Autodesk Inventor part; units mm, degrees
ref_plane "YZ Plane" through (0, 0, 0) normal (1, 0, 0) x (0, 1, 0)
ref_plane "XZ Plane" through (0, 0, 0) normal (0, 1, 0) x (-1, 0, 0)
ref_plane "XY Plane" through (0, 0, 0) normal (0, 0, 1) x (1, 0, 0)
sketch "Sketch1" plane through (0, 0, 0) normal (0, 1, 0) x (-1, 0, 0)
  line L0 (-10.16, 10.16) -> (10.16, 10.16)
  line L1 (10.16, 10.16) -> (10.16, -10.16)
  line L2 (-10.16, -10.16) -> (-10.16, 10.16)
  circle A0 centre (6.9088, -6.9148) radius 1.9304
  circle A1 centre (6.9088, 6.9088) radius 1.9304
  circle A2 centre (-6.9088, 6.9088) radius 1.9304
  circle A3 centre (-6.9088, -6.9148) radius 1.9304
  line L3 (-5.715, -10.16) -> (-5.715, -20.574)
  line L4 (-5.715, -20.574) -> (5.715, -20.574)
  line L5 (5.715, -20.574) -> (5.715, -10.16)
  line L6 (10.16, -10.16) -> (5.715, -10.16)
  line L7 (-5.715, -10.16) -> (-10.16, -10.16)
  point P0 (0, 0)
  dimension "d0" = 20.32
  dimension "d2" = 10.16
  dimension "d3" = 10.16
  dimension "d4" = 3.8608
  dimension "d5" = 6.9148
  dimension "d6" = 6.9088
  dimension "d7" = 3.8608
  dimension "d8" = 6.9088
  dimension "d9" = 6.9088
  dimension "d10" = 3.8608
  dimension "d11" = 6.9088
  dimension "d12" = 6.9088
  dimension "d13" = 3.8608
  dimension "d14" = 11.43
  dimension "d16" = 5.715
extrude "Extrusion1" add sketch "Sketch1" along normal blind 6.985
sketch "Sketch2" plane through (-5.715, 0, -20.574) normal (-1, 0, 0) x (0, 0, 1)
  circle A0 centre (5.08, 3.4925) radius 4.6609 construction
  line L0 (10.414, 0) -> (0, 0)
  line L1 (0, 0) -> (0, 6.985)
  line L2 (9.7409, 3.4925) -> (7.4105, -0.544)
  line L3 (7.4105, -0.544) -> (2.7496, -0.544)
  line L4 (2.7496, -0.544) -> (0.4191, 3.4925)
  line L5 (0.4191, 3.4925) -> (2.7495, 7.529)
  line L6 (2.7495, 7.529) -> (7.4104, 7.529)
  line L7 (7.4104, 7.529) -> (9.7409, 3.4925)
  point P0 (20.574, 0)
  dimension "d19" = 9.3218
  dimension "d20" = 3.4925
  dimension "d21" = 5.08
extrude "Extrusion2" cut sketch "Sketch2" against normal blind 3.81
sketch "Sketch3" plane through (5.715, 0, -10.16) normal (1, 0, 0) x (0, 0, -1)
  circle A0 centre (5.334, 3.4925) radius 1.9304
  line L0 (10.414, 0) -> (10.414, 6.985)
  line L1 (0, 6.985) -> (10.414, 6.985)
  point P0 (-10.16, 0)
  dimension "d24" = 3.8608
  dimension "d25" = 5.08
  dimension "d26" = 3.4925
extrude "Extrusion3" cut sketch "Sketch3" against normal through all
sketch "Sketch4" plane through (0, 6.985, 0) normal (0, 1, 0) x (1, 0, 0)
  circle A0 centre (0, 0) radius 6.35
  dimension "d29" = 12.7
extrude "Extrusion4" add sketch "Sketch4" along normal blind 2.54
sketch "Sketch5" plane through (0, 9.525, 0) normal (0, 1, 0) x (1, 0, 0)
  arc A0 (2.0472, -2.5908) -> (-2.0472, -2.5908) centre (0, 0) ccw
  line L0 (-2.0472, -2.5908) -> (2.0472, -2.5908)
  dimension "d32" = 6.604
  dimension "d33" = 2.5908
fillet "Fillet1" radius 3.3782 4 edges at (10.16, 3.4925, 10.16) (10.16, 3.4925, -10.16) (-10.16, 3.4925, 10.16) (-10.16, 3.4925, -10.16)
extrude "Extrusion5" cut sketch "Sketch5" against normal through all
sketch "Sketch6" plane through (0, 9.525, 0) normal (0, 1, 0) x (1, 0, 0)
  line L0 (-5.715, 20.574) -> (5.715, 20.574)
  line L1 (0.635, 0) -> (0.635, 20.574)
  line L2 (0.635, 20.574) -> (-0.635, 20.574)
  line L3 (-0.635, 20.574) -> (-0.635, 0)
  line L4 (-0.635, -20.574) -> (0.635, 20.574) construction
  line L5 (0.635, -20.574) -> (-0.635, 20.574) construction
  line L6 (-0.635, 0) -> (0.635, 0)
  point P0 (0, 0)
  dimension "d37" = 1.27
extrude "Extrusion6" cut sketch "Sketch6" against normal through all
properties part number "clamping hub 1_4 D a"
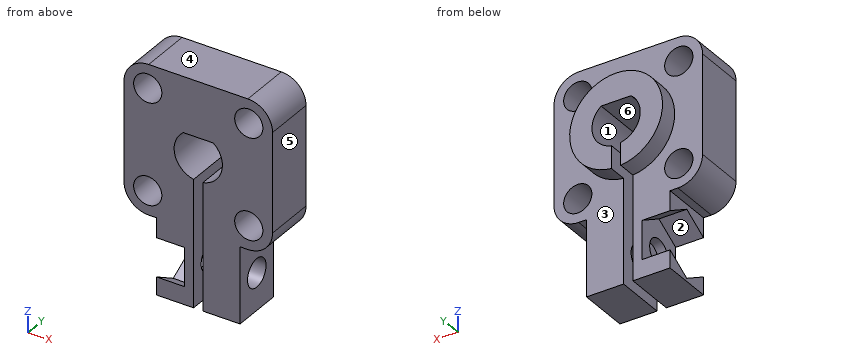
Check sheet for the modelled part. Datum: model origin and axes. Units: mm. Face numbers are marked on the shaded views. A direction names the side the tool comes from. Round coordinates to 2 decimals unless told otherwise and drop trailing zeros. Loops run counter-clockwise (first coordinate to the right, second up) from the corner with the lowest first, then second, coordinate; pieces in that order, holes last. Notation, with made-up numbers: (8, -18) -> (39, -18) arc R9 ccw to (39, -12) -> close; hole circle Ø10 at (-35.5, -34.75). An arc over 180 degrees is marked (long way). Put each result on its own line as item: value. Start each with the question number.
1. Draft check along Z on the marked faces 4, 5 and 6. Enter one of: +Z half, -Z half, draft (parallel to the pull), parting line (faces both ways), or undercut.
2. Section check A-A (y = 5). Give the number of separate pieces and of enclosed holes in the cut face, plus the area to 3 significant figures.
3. Section check B-B (z = 0). Enter the section's corners in (x, y) (3 decimals), plus the area to 3 significant figures.
4. Section check C-C (x = 0). Enter the section's corners in (y, z) (3 decimals).
5. Gauge pin test, flat ends, axial feed: pin 1 (3.5 mm diameter, centred on y = 3.5, z = -15, fed in from +X) (3 decimals); pin 2 (1.2 mm diameter, centred on x = -6.5, y = 5, fed in from -Z); pin 3 (2.5 mm diameter, centred on y = 2.5, z = -19.5, fed in from -X) (3 decimals). Record the tip position at first contact, or that the pin passes through.
6. Section check D-D (z = -6). Enter the section's corners in (x, y) (3 decimals), plus the area to 3 significant figures.
7. Scan lines: probe 1 along X at (y, z) = (5, -12.5) (3 decimals); probe 2 along Z at (x, y) = (-2.75, 0.5); probe 3 along X at (y, z) = (4, 5.5). Record each from-to range of solid material in increasing order.
8. Access from +Z, -Z, +X, -X, +Y, -Y to the whole of each face (thin tool, end or side, straight path). Record for the marked faces 1, 2 and 3.
Findings:
1. face 4: +Z half
1. face 5: draft
1. face 6: undercut
2. separate pieces: 3
2. enclosed holes: 4
2. area: 377 mm^2
3. outline: (-10.16, 0) -> (-3.302, 0) -> (-3.302, 9.525) -> (-6.35, 9.525) -> (-6.35, 6.985) -> (-10.16, 6.985) -> close; (3.302, 0) -> (10.16, 0) -> (10.16, 6.985) -> (6.35, 6.985) -> (6.35, 9.525) -> (3.302, 9.525) -> close
3. area: 111 mm^2
4. outline: (0, 2.591) -> (9.525, 2.591) -> (9.525, 6.35) -> (6.985, 6.35) -> (6.985, 10.16) -> (0, 10.16) -> close
5. pin 1: stops at x = 5.715
5. pin 2: stops at z = -10.16
5. pin 3: stops at x = -5.715
6. outline: (-10.16, 0) -> (-8.609, 0) -> (-8.609, 6.985) -> (-10.16, 6.985) -> close; (-5.209, 0) -> (-0.635, 0) -> (-0.635, 9.525) -> (-2.079, 9.525) -> (-2.079, 6.985) -> (-5.209, 6.985) -> close; (0.635, 0) -> (5.209, 0) -> (5.209, 6.985) -> (2.079, 6.985) -> (2.079, 9.525) -> (0.635, 9.525) -> close; (8.609, 0) -> (10.16, 0) -> (10.16, 6.985) -> (8.609, 6.985) -> close
6. area: 92.9 mm^2
7. probe 1: x = -1.905 to -0.635, 0.635 to 5.715
7. probe 2: z = -20.57 to -18.43, -12.56 to -1.83, 1.83 to 10.16
7. probe 3: x = -10.16 to -8.23, -5.59 to 5.59, 8.23 to 10.16
8. face 1: +Y, -Y
8. face 2: -X
8. face 3: +Y
